```python
from build123d import *
from build123d import SkipClean  # not in build123d's __all__

# Parameters (mm, degrees)
F1_DEPTH    = 2
F2_W        = 33
F2_H        = 5
F3_DEPTH    = 5
F6_R        = 1.5
F7_DEPTH    = 42
F8_T1_DEPTH = 54.6506350946
F10_DEPTH   = 39.001


# Not quite as in the source:
# - a fillet or chamfer that OpenCascade refuses, or shapes differently, is made with other operations: its cross-section is extruded or revolved along the edge and cut away or added


with BuildPart() as f1:
    # F0 (on Top) → F1 (new body)
    with BuildSketch(Plane.XY):
        with BuildLine():
            Line((-21.5, -15.5), (21.5, -15.5))
            ThreePointArc((21.5, -15.5), (22.2071067812, -15.2071067812), (22.5, -14.5))
            Line((22.5, -14.5), (22.5, 14.5))
            ThreePointArc((22.5, 14.5), (22.2071067812, 15.2071067812), (21.5, 15.5))
            Line((21.5, 15.5), (17.5, 15.5))
            ThreePointArc((17.5, 15.5), (16.7928932188, 15.2071067812), (16.5, 14.5))
            Line((16.5, 14.5), (16.5, -9.5))
            Line((16.5, -9.5), (-16.5, -9.5))
            Line((-16.5, -9.5), (-16.5, 14.5))
            ThreePointArc((-16.5, 14.5), (-16.7928932188, 15.2071067812), (-17.5, 15.5))
            Line((-17.5, 15.5), (-21.5, 15.5))
            ThreePointArc((-21.5, 15.5), (-22.2071067812, 15.2071067812), (-22.5, 14.5))
            Line((-22.5, 14.5), (-22.5, -14.5))
            ThreePointArc((-22.5, -14.5), (-22.2071067812, -15.2071067812), (-21.5, -15.5))
        make_face()
    extrude(amount=F1_DEPTH)

    # F2 (on face) → F3 (join)
    with BuildSketch(Plane.XY.offset(2)):
        with Locations((0, -12)):
            Rectangle(F2_W, F2_H)
    extrude(amount=F3_DEPTH)

    # F6 (on offset) → F7 (join, through all)
    with BuildSketch(Plane.YZ.offset(21)):
        with Locations((-13.5, 7)):
            Circle(F6_R)
    extrude(amount=-F7_DEPTH)

    # F8: fillet of radius 5 on 1 edges, made by hand

    # F8_s2 → F8_t1 (cut)
    with BuildSketch(Plane.YZ.offset(-27.3253175473)):
        with BuildLine():
            ThreePointArc((-9.5, 2.6698729811), (-10.1698729811, 5.1698729811), (-12, 7))
            Line((-12, 7), (-9.5, 7))
            Line((-9.5, 7), (-9.5, 2.6698729811))
        make_face()
    extrude(amount=F8_T1_DEPTH, mode=Mode.SUBTRACT)

    # F9 (on face) → F10 (cut, through all)
    with BuildSketch(Plane.YZ.offset(16.5)):
        with BuildLine():
            ThreePointArc((-13.6298629558, 5.5056320357), (-14.0954446994, 5.6232481669), (-14.5, 5.8819660113))
            Line((-14.5, 5.8819660112), (-14.5, 2))
            Line((-14.5, 2), (-12, 2))
            ThreePointArc((-12, 2), (-12.1749548088, 4.0503584453), (-13.6298629558, 5.5056320357))
        make_face()
    with SkipClean():  # cleaning this boolean's faces spoils the solid; the shape is the same uncleaned
        extrude(amount=-F10_DEPTH, mode=Mode.SUBTRACT)


solid = f1.part
```
Check sheet for the modelled part. Datum: model origin and axes. Units: mm. A direction names the side the tool comes from. Give positions to 0.01 mm unless a question says otherwise; leave off trailing zeros. Write each loop counter-clockwise with the first axis right and the second up, starting at its lowest first coordinate (ties: lowest second). Pieces come first, ordered by that corner, then holes.
Item 1: Access from +Z, -Z, +X, -X, +Y, -Y to the whole of each face (thin tool, end or side, straight path). Record for faces 1 (the face through (16.801, 15.215, 0.986)), 2 (the face through (16.5, -11, 4)), 3 (the face through (-16.5, -11, 4)).
Item 2: Cross-section at B-B (y = 5). Enter the section's corners in (x, z), and give its area (3 significant figures).
Item 3: Scan lines: L1, parallel to Z at x = -17, y = 1.5; L2, parallel to Y at x = -11.5, z = 1.5; L3, parallel to X at y = -10.5, z = 4.5. Record each from-to range of solid material in increasing order.
Item 4: Gauge pin test, flat ends, axial feed: pin 1 (6.5 mm diameter, centred on x = -19.5, y = 5, fed in from +Z); pin 2 (2 mm diameter, centred on x = 6.5, z = 1.5, fed in from +Y); pin 3 (1.5 mm diameter, centred on y = -13, z = 7, fed in from -X). Record the tip position at first contact, or that the pin passes through.
Item 5: Cross-section at A-A (z = 1.25). Enter the section's corners in (x, y).
Item 6: Cross-section at D-D (x = 11). Enter the section's corners in (y, z).
Item 7: Cross-section at C-C (x = -19). Enter the section's corners in (y, z).
Item 8: Draft check along X on faces 4 (the face through (16.5, 3, 1)), 5 (the face through (22.199, -15.215, 0.986)), 6 (the face through (-19, 15.5, 1)), 7 (the face through (-21, -14, 7)). Enter one of: released by +X, released by -X, zero draft, split by the parting line, or undercut.
Report:
1. face 1: +Z, -Z, +Y
1. face 2: +X, +Y
1. face 3: -X, +Y
2. outline: (-22.5, 0) - (-16.5, 0) - (-16.5, 2) - (-22.5, 2) - close; (16.5, 0) - (22.5, 0) - (22.5, 2) - (16.5, 2) - close
2. area: 24.0 mm2
3. L1: z = 0 to 2
3. L2: y = -15.5 to -9.5
3. L3: x = -16.5 to 16.5
4. pin 1: stops at z = 2
4. pin 2: stops at y = -9.5
4. pin 3: stops at x = -21
5. outline: (-22.5, -14.5) arc R1 ccw to (-21.5, -15.5) - (21.5, -15.5) arc R1 ccw to (22.5, -14.5) - (22.5, 14.5) arc R1 ccw to (21.5, 15.5) - (17.5, 15.5) arc R1 ccw to (16.5, 14.5) - (16.5, -9.5) - (-16.5, -9.5) - (-16.5, 14.5) arc R1 ccw to (-17.5, 15.5) - (-21.5, 15.5) arc R1 ccw to (-22.5, 14.5) - close
6. outline: (-15.5, 0) - (-9.5, 0) - (-9.5, 2.67) arc R5 ccw to (-12, 7) arc R1.5 ccw (long way) to (-13.63, 5.51) arc R3 cw to (-12, 2) - (-15.5, 2) - close
7. outline: (-15.5, 0) - (15.5, 0) - (15.5, 2) - (-15.5, 2) - close; circle Ø3 at (-13.5, 7)
8. face 4: undercut
8. face 5: released by +X
8. face 6: zero draft
8. face 7: released by -X
